```python
from build123d import *

# Parameters (mm, degrees)
F0_W     = 38.1
F0_H     = 25.4
F0_R     = 4.1656
F1_DEPTH = 12.7
F2_R     = 3.175
F3_DEPTH = 19.05
F4_R     = 1.5875
F5_DEPTH = 12.7


with BuildPart() as f1:
    # F0 (on Top) → F1 (new body)
    with BuildSketch(Plane.XY):
        with Locations((-8.1788, 0)):
            Rectangle(F0_W, F0_H)
        Circle(F0_R, mode=Mode.SUBTRACT)
    extrude(amount=-F1_DEPTH)

    # F2 (on face) → F3 (cut)
    with BuildSketch(Plane(origin=(-27.2288, 0, 0), x_dir=(0, -1, 0), z_dir=(-1, 0, 0))):
        with Locations((0, -6.35)):
            Circle(F2_R)
    extrude(amount=-F3_DEPTH, mode=Mode.SUBTRACT)

    # F4 (on face) → F5 (cut)
    with BuildSketch(Plane.YZ.offset(10.8712)):
        with Locations((0, -6.35)):
            Circle(F4_R)
    extrude(amount=-F5_DEPTH, mode=Mode.SUBTRACT)


solid = f1.part
```
Input: part model. Units: mm. Frame: model coordinates. A direction names the side the tool comes from. Coordinates: 2 decimals unless noted, no trailing zeros. Write each loop counter-clockwise with the first axis right and the second up, starting at its lowest first coordinate (ties: lowest second). Pieces come first, ordered by that corner, then holes. Notation, with made-up numbers: (73.25, 10) -> (104.25, 10) arc R28 ccw to (104.25, 30) -> close; hole circle Ø7 at (-30.5, 16.25). An arc over 180 degrees is marked (long way). Answer as a JSON object with one key per item and string values.
1. Section B-B on y = 0. Return the cut outline in (x, z) (1 decimal).
Result set:
{"outline": "(-27.2, -12.7) -> (-4.2, -12.7) -> (-4.2, 0) -> (-27.2, 0) -> (-27.2, -3.2) -> (-8.2, -3.2) -> (-8.2, -9.5) -> (-27.2, -9.5) -> close; (4.2, -12.7) -> (10.9, -12.7) -> (10.9, -7.9) -> (4.2, -7.9) -> close; (4.2, -4.8) -> (10.9, -4.8) -> (10.9, 0) -> (4.2, 0) -> close"}
2. Mould query, pull axis Z, two halves, no side actions, for faces 1 (the face through (-8, 0, 0)), 2 (the face through (7.41, -0.34, -7.9)), 3 (the face through (-8, 0, -12.7)), 4 (the face through (10.871, 3, -6)). Classes: released by +Z, released by -Z, zero draft, split by the parting line, or undercut.
Result set:
{"face 1": "released by +Z", "face 2": "undercut", "face 3": "released by -Z", "face 4": "zero draft"}
3. Section D-D on x = -15.5. Return the cut outline in (y, z) (3 decimals), then the cut area to 3 significant figures.
Result set:
{"outline": "(-12.7, -12.7) -> (12.7, -12.7) -> (12.7, 0) -> (-12.7, 0) -> close; hole circle Ø6.35 at (0, -6.35)", "area": "291 mm2"}
4. Access query for faces 5 (the face through (-8.179, 0, -6)), 6 (the face through (-8, 12.7, -6)). Directions: +Z, -Z, +X, -X, +Y, -Y. A direction counts if a zero-diameter tool reaches every point of the face in a straight line with its end or side. Return the directions, or none.
Result set:
{"face 5": "-X", "face 6": "+Z, -Z, +X, -X, +Y"}
5. First-contact query: P1, Ø7.5, axis at y = 0, z = -6.35, coming from the +X side; P2, Ø1.9, axis at y = -1, z = -5, coming from the -X side; P3, Ø1.9, axis at y = 0, z = -6.35, coming from the +X side. Flat tips, straight axial feed; report the tip coordinate or a pass-through.
Result set:
{"P1": "stops at x = 10.87", "P2": "stops at x = -8.18", "P3": "stops at x = -4.06"}
6. Material intervals for line 1 (Y direction, x = 8.5, z = -6.35); line 2 (Y direction, x = 0, z = -7.75); line 3 (Z direction, x = 8.75, y = 0), sorted ascending. Write a range as from..to.
Result set:
{"line 1": "y = -12.7..-1.59, 1.59..12.7", "line 2": "y = -12.7..-4.17, 4.17..12.7", "line 3": "z = -12.7..-7.94, -4.76..0"}
7. Section A-A on z = -2.5. Return the cut outline in (x, y), then the cut area to 3 significant figures.
Result set:
{"outline": "(-27.23, -12.7) -> (10.87, -12.7) -> (10.87, 12.7) -> (-27.23, 12.7) -> close; hole circle Ø8.33 at (0, 0)", "area": "913 mm2"}
8. Section C-C on x = 0. Return the cut outline in (y, z), then the cut area to 3 significant figures.
Result set:
{"outline": "(-12.7, -12.7) -> (-4.17, -12.7) -> (-4.17, 0) -> (-12.7, 0) -> close; (4.17, -12.7) -> (12.7, -12.7) -> (12.7, 0) -> (4.17, 0) -> close", "area": "217 mm2"}
